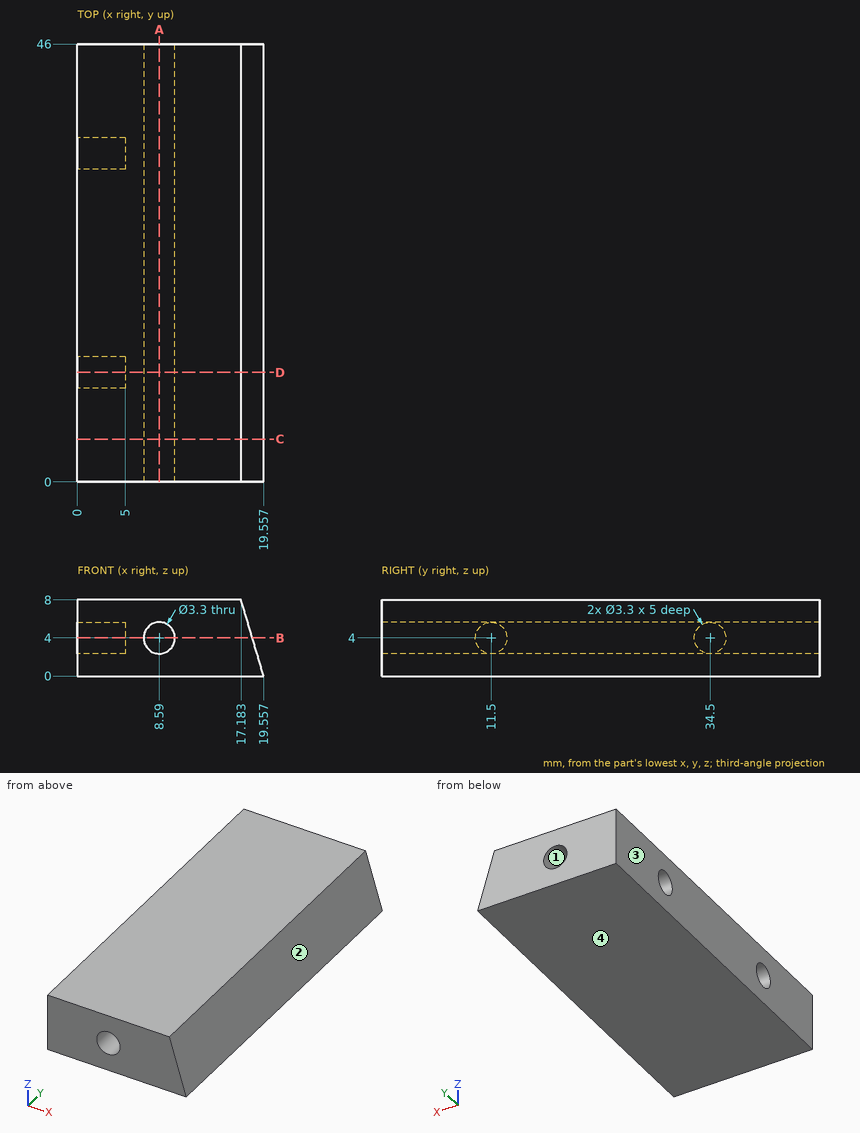
Answer from the drawing. Dimensions are ordinates in mm from the lowest x, y and z of the part. Give positions to 0.01 mm unless a question says otherwise; leave off trailing zeros. Loops run counter-clockwise (first coordinate to the right, second up) from the corner with the lowest first, then second, coordinate; pieces in that order, holes last. Notation, with made-up numbers: M 42.25,-15 L 67.25,-15 A30 ccw 67.25,16 Z; hole C 4,12.25 d2. An arc over 180 degrees is marked long. One line per item, written item: value.
Q1. Determine the mould class of the marked faces 1, 2, 3 and 4 for opening direction Z: +Z half, -Z half, draft (parallel to the pull), parting line (faces both ways), or undercut.
Working result:
face 1: undercut
face 2: +Z half
face 3: draft
face 4: -Z half
Q2. Flat-ended cylindrical pins translate along their axes: P1, Ø2.5, axis at y = 11.5, z = 4, coming from the -X side; P2, Ø4, axis at y = 25, z = 4, coming from the +X side. Find the tip coordinate at first contact, or state that the pin passes through.
Working result:
P1: stops at x = 5
P2: stops at x = 18.96
Q3. Find the intervals of material crossed by line 1 (Y direction, x = 3.2, z = 4); line 2 (Z direction, x = 8.59, y = 28); line 3 (Y direction, x = 2.5, z = 5), in increasing order. Write a range as from..to.
Working result:
line 1: y = 0..9.85, 13.15..32.85, 36.15..46
line 2: z = 0..2.35, 5.65..8
line 3: y = 0..10.19, 12.81..33.19, 35.81..46
Q4. A cutting plane is placed at D-D on y = 11.5. Determine the outline of the cut face in (x, z).
Working result:
outline: M 0,0 L 19.56,0 L 17.18,8 L 0,8 L 0,5.65 L 5,5.65 L 5,2.35 L 0,2.35 Z; hole C 8.59,4 d3.3
Q5. A cutting plane is placed at C-C on y = 4.5. Determine the outline of the cut face in (x, z).
Working result:
outline: M 0,0 L 19.56,0 L 17.18,8 L 0,8 Z; hole C 8.59,4 d3.3
Q6. A cutting plane is placed at A-A on x = 8.59. Determine the outline of the cut face in (y, z), then the cut area to 3 significant figures.
Working result:
outline: M 0,0 L 46,0 L 46,2.35 L 0,2.35 Z; M 0,5.65 L 46,5.65 L 46,8 L 0,8 Z
area: 216 mm^2
Q7. A cutting plane is placed at B-B on z = 4. Determine the outline of the cut face in (x, y), then the cut area to 3 significant figures.
Working result:
outline: M 0,0 L 6.94,0 L 6.94,46 L 0,46 L 0,36.15 L 5,36.15 L 5,32.85 L 0,32.85 L 0,13.15 L 5,13.15 L 5,9.85 L 0,9.85 Z; M 10.24,0 L 18.37,0 L 18.37,46 L 10.24,46 Z
area: 660 mm^2
